from build123d import *

# Parameters (mm, degrees)
EXTRUDE_1_DEPTH     = 17.5
SKETCH_2_R          = 7.5
CUT_EXTRUDE_1_DEPTH = 73.844011422
SKETCH_3_R          = 12
CUT_EXTRUDE_2_DEPTH = 15
SKETCH_4_R          = 23.5
CUT_EXTRUDE_3_DEPTH = 9


with BuildPart() as part:
    # 草图1 → 凸台-拉伸1 (new, symmetric)
    with BuildSketch(Plane.XY):
        with BuildLine():
            Line((21.5, -25), (50, -25))
            Line((50, -25), (50, 25))
            Line((50, 25), (-50, 25))
            Line((-50, 25), (-50, -25))
            Line((-50, -25), (-21.5, -25))
            ThreePointArc((-21.5, -25), (0, -3.5), (21.5, -25))
        make_face()
    extrude(amount=EXTRUDE_1_DEPTH, both=True)

    # 草图2 → 切除-拉伸1 (cut, through all)
    with BuildSketch(Plane(origin=(0, 25, 0), x_dir=(1, 0, 0), z_dir=(0, 1, 0))):
        with Locations(Location((-35, 0, 0), (0, 0, 270))):
            Circle(SKETCH_2_R)
        with Locations(Location((35, 0, 0), (0, 0, 270))):
            Circle(SKETCH_2_R)
    extrude(amount=-CUT_EXTRUDE_1_DEPTH, mode=Mode.SUBTRACT)

    # 草图3 → 切除-拉伸2 (cut)
    with BuildSketch(Plane(origin=(0, 25, 0), x_dir=(1, 0, 0), z_dir=(0, 1, 0))):
        with Locations(Location((-35, 0, 0), (0, 0, 270))):
            Circle(SKETCH_3_R)
        with Locations(Location((35, 0, 0), (0, 0, 270))):
            Circle(SKETCH_3_R)
    extrude(amount=-CUT_EXTRUDE_2_DEPTH, mode=Mode.SUBTRACT)

    # 草图4 → 切除-拉伸3 (cut, symmetric)
    with BuildSketch(Plane.XY):
        with Locations((0, -25)):
            Circle(SKETCH_4_R)
    extrude(amount=CUT_EXTRUDE_3_DEPTH, both=True, mode=Mode.SUBTRACT)


solid = part.part
The model under review builds one solid part; all positions refer to its coordinate system, in mm. A direction names the side the tool comes from. Coordinates: 2 decimals unless noted, no trailing zeros. Loops run counter-clockwise (first coordinate to the right, second up) from the corner with the lowest first, then second, coordinate; pieces in that order, holes last. Notation, with made-up numbers: M 50.5,-13.75 L 62.5,-13.75 A18 cw 62.5,-7.75 Z; hole C 50,10 d3. An arc over 180 degrees is marked long. Put each result on its own line as item: value. Start each with the question number.
Q1. Add section A-A (z = 0). Write out the cut boundary in (x, y).
Q2. The part is to be moulded in two halves that separate along Z. For faces 4 (the flat face through (-1, 0, 17.5)), 5 (the cylindrical face through (0.517, -1.506, 0.126)), 6 (the flat face through (42, -25, 4)), say which applies: +Z half, -Z half, draft (parallel to the pull), parting line (faces both ways), or undercut.
Q3. For faces 1 (the flat face through (-3.6, -3.6, 9)), 2 (the cylindrical face through (-0.473, -3.505, -13.19)), 3 (the flat face through (-40, 10, -6)), list the 3-axis set-ups (+Z, -Z, +X, -X, +Y, -Y) from which the entire face can be reached by the end or side of a thin tool; tool diameter is ignored.
Q4. Clearance check with flat-ended pins moving along their axes: pin 1 (12 mm diameter, centred on x = 11, y = -17, fed in from -Z); pin 2 (1.5 mm diameter, centred on x = -0.5, z = 0.5, fed in from -Y). State where each tip first meets the part, or that it passes through.
Q5. Add section D-D (x = 0). Write out the cut boundary in (y, z), and give its area (4 significant figures).
Q6. Add section C-C (y = 8). Write out the cut boundary in (x, z), and give its area (3 significant figures).
Q7. Add section B-B (x = 35). Write out the cut boundary in (y, z).
Q8. Wall thickness on line 1 (X direction, y = 17, z = 0); line 2 (X direction, y = -1, z = 0); line 3 (Z direction, x = 35.5, y = -13): over which ranges is each line inside the solid? List them lowest first.
Answers:
1. outline: M -50,-25 L -42.5,-25 L -42.5,10 L -47,10 L -47,25 L -50,25 Z; M -27.5,-25 L -23.5,-25 A23.5 cw 23.5,-25 L 27.5,-25 L 27.5,10 L 23,10 L 23,25 L -23,25 L -23,10 L -27.5,10 Z; M 42.5,-25 L 50,-25 L 50,25 L 47,25 L 47,10 L 42.5,10 Z
2. face 4: +Z half
2. face 5: undercut
2. face 6: draft
3. face 1: -Y
3. face 2: +Z, -Z, -Y
3. face 3: +Y
4. pin 1: passes through
4. pin 2: stops at y = -1.53
5. outline: M -3.5,-17.5 L 25,-17.5 L 25,17.5 L -3.5,17.5 L -3.5,9 L -1.5,9 L -1.5,-9 L -3.5,-9 Z
5. area: 961.5 mm^2
6. outline: M -50,-17.5 L 50,-17.5 L 50,17.5 L -50,17.5 Z; hole C -35,0 d15; hole C 35,0 d15
6. area: 3,150 mm^2
7. outline: M -25,-17.5 L 25,-17.5 L 25,-12 L 10,-12 L 10,-7.5 L -25,-7.5 Z; M -25,7.5 L 10,7.5 L 10,12 L 25,12 L 25,17.5 L -25,17.5 Z
8. line 1: x = -50 to -47, -23 to 23, 47 to 50
8. line 2: x = -50 to -42.5, -27.5 to 27.5, 42.5 to 50
8. line 3: z = -17.5 to -7.48, 7.48 to 17.5
